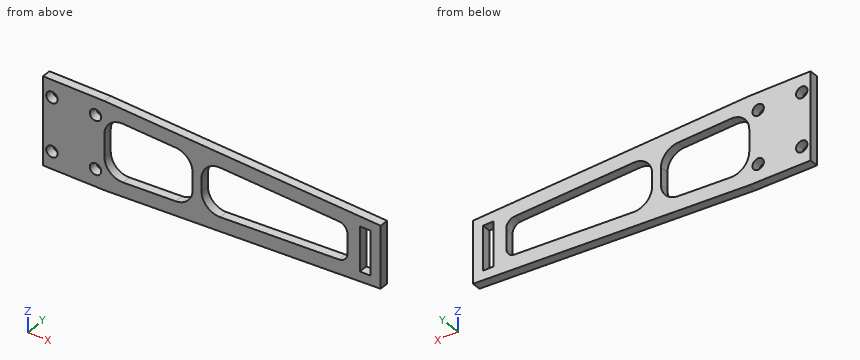
```python
from build123d import *

# Parameters (mm, degrees)
SKETCH1_W           = 34.5
SKETCH1_H           = 49.5
BOSS_EXTRUDE1_DEPTH = 5
SKETCH2_R           = 3.2
CUT_EXTRUDE1_DEPTH  = 5
SKETCH3_W           = 6
SKETCH3_H           = 25
BOSS_EXTRUDE2_DEPTH = 5
FILLET1_R           = 10
FILLET2_R           = 5


with BuildPart() as part:
    # Sketch1 → Boss-Extrude1 (new body)
    with BuildSketch(Plane(origin=(0, 0, 0), x_dir=(1, 0, 0), z_dir=(0, 1, 0))):
        with Locations((17.25, 24.75)):
            Rectangle(SKETCH1_W, SKETCH1_H)
    extrude(amount=BOSS_EXTRUDE1_DEPTH)

    # Sketch2 → Cut-Extrude1 (cut)
    with BuildSketch(Plane(origin=(0, 5, 0), x_dir=(1, 0, 0), z_dir=(0, 1, 0))):
        with Locations(Location((5, 39.75, 0), (0, 0, 270))):
            Circle(SKETCH2_R)
        with Locations(Location((5, 9.75, 0), (0, 0, 90))):
            Circle(SKETCH2_R)
        with Locations(Location((29.5, 9.75, 0), (0, 0, 270))):
            Circle(SKETCH2_R)
        with Locations(Location((29.5, 39.75, 0), (0, 0, 90))):
            Circle(SKETCH2_R)
    extrude(amount=-CUT_EXTRUDE1_DEPTH, mode=Mode.SUBTRACT)

    # Sketch3 → Boss-Extrude2 (add)
    with BuildSketch(Plane(origin=(0, 5, 0), x_dir=(1, 0, 0), z_dir=(0, 1, 0))):
        Polygon((189.75, 42.25), (34.5, 49.5), (34.5, 41.491281612), (84.094915791, 39.175254948), (84.094915791, 10.324745052), (34.5, 8.008718388), (34.5, 0), (189.75, 7.25), align=None)
        Polygon((171.053500921, 14.385612956), (89.094915791, 10.558239416), (89.094915791, 38.941760584), (171.053500921, 35.114387044), align=None, mode=Mode.SUBTRACT)
        with Locations((181.13, 24.75)):
            Rectangle(SKETCH3_W, SKETCH3_H, mode=Mode.SUBTRACT)
    extrude(amount=-BOSS_EXTRUDE2_DEPTH)

    # Fillet1
    fillet1_edges = [part.edges().sort_by_distance(p)[0] for p in [
        (34.5, 2.5, -8.008718388),
        (84.094915791, 2.5, -10.324745052),
        (84.094915791, 2.5, -39.175254948),
        (34.5, 2.5, -41.491281612),
        (89.094915791, 2.5, -38.941760584),
        (89.094915791, 2.5, -10.558239416),
    ]]
    fillet(fillet1_edges, radius=FILLET1_R)

    # Fillet2
    fillet2_edges = [part.edges().sort_by_distance(p)[0] for p in [
        (171.053500921, 2.5, -35.114387044),
        (171.053500921, 2.5, -14.385612956),
    ]]
    fillet(fillet2_edges, radius=FILLET2_R)


solid = part.part
```
The listing builds one solid part. Answer for the finished solid, in the listing's coordinates (mm). Give positions to 0.01 mm unless a question says otherwise; leave off trailing zeros. Loops run counter-clockwise (first coordinate to the right, second up) from the corner with the lowest first, then second, coordinate; pieces in that order, holes last. Notation, with made-up numbers: (71, -1) - (91, -1) arc R28 ccw to (91, 24) - close; hole circle Ø7 at (40.25, 29.25). An arc over 180 degrees is marked (long way). Answer as CSV lines item,"result". Start each with the question number.
Item 1: A cutting plane is placed at C-C on y = 1.6. Count the separate pieces of the cut face and the enclosed holes in it, then the cut area to 3 significant figures.
Item 2: This flat-tipped pin is pushed along its axis until it touches: pin 1 (5 mm diameter, centred on x = 29.5, z = -39.75, fed in from +Y). Where does it stop, or does it pass through?
Item 3: A cutting plane is placed at D-D on x = 147. Determine the outline of the cut face in (y, z).
Item 4: A cutting plane is placed at B-B on x = 5. Determine the outline of the cut face in (y, z), then the cut area to 4 significant figures.
Item 5: A cutting plane is placed at A-A on z = -25. Determine the outline of the cut face in (x, y), then the cut area to 3 significant figures.
Item 6: Find the intervals of material crossed by line 1 (X direction, y = 3.9, z = -24.5); line 2 (X direction, y = 3.5, z = -15); line 3 (Z direction, x = 167, y = 2.5), in increasing order. Write a range as from..to.
Found:
1,separate pieces,"1"
1,enclosed holes,"7"
1,area,"4,570 mm^2"
2,pin 1,"passes through"
3,outline,"(0, -44.25) - (5, -44.25) - (5, -36.24) - (0, -36.24) - close; (0, -13.26) - (5, -13.26) - (5, -5.25) - (0, -5.25) - close"
4,outline,"(0, -49.5) - (5, -49.5) - (5, -42.95) - (0, -42.95) - close; (0, -36.55) - (5, -36.55) - (5, -12.95) - (0, -12.95) - close; (0, -6.55) - (5, -6.55) - (5, 0) - (0, 0) - close"
4,area,"183.5 mm^2"
5,outline,"(0, 0) - (34.5, 0) - (34.5, 5) - (0, 5) - close; (84.09, 0) - (89.09, 0) - (89.09, 5) - (84.09, 5) - close; (171.05, 0) - (178.13, 0) - (178.13, 5) - (171.05, 5) - close; (184.13, 0) - (189.75, 0) - (189.75, 5) - (184.13, 5) - close"
5,area,"261 mm^2"
6,line 1,"x = 0..34.5, 84.09..89.09, 171.05..178.13, 184.13..189.75"
6,line 2,"x = 0..35.13, 82.83..91.12, 168.83..178.13, 184.13..189.75"
6,line 3,"z = -43.31..-35.25, -14.25..-6.19"
